from build123d import *

# Parameters (mm, degrees)
SKETCH_1_W             = 40
SKETCH_1_H             = 62
EXTRUDE_1_DEPTH        = 1
SKETCH_3_W             = 27.6
SKETCH_3_H             = 27.6
SKETCH_3_W_2           = 6.7
SKETCH_3_H_2           = 6.7
CUT_EXTRUDE_1_DEPTH    = 37.905284174
EXTRUDE_2_DEPTH        = 1
SKETCH_8_W             = 40
SKETCH_8_H             = 1
EXTRUDE_5_DEPTH        = 1
SKETCH_10_W            = 0.6
SKETCH_10_H            = 2
EXTRUDE_6_DEPTH        = 9
SKETCH_11_W            = 38.8
SKETCH_11_H            = 1
EXTRUDE_7_DEPTH        = 9
CUT_EXTRUDE_2_REACH    = 68.708
SKETCH_13_W            = 7.2
SKETCH_13_H            = 2.2
SKETCH_13_W_2          = 9.4
SKETCH_13_H_2          = 3.8
SKETCH_13_W_3          = 15
SKETCH_13_H_3          = 2.4
CUT_EXTRUDE_3_DEPTH    = 10
SKETCH_15_W            = 0.891909811
SKETCH_15_H            = 2.2
EXTRUDE_8_DEPTH        = 2.2
CUT_EXTRUDE_4_REACH    = 41.79
FILLET_1_R             = 0.5
FILLET_1_OF_MIRROR_1_R = 0.5


with BuildPart() as part:
    # 草图1 → 凸台-拉伸1 (new body)
    with BuildSketch(Plane.XY):
        Rectangle(SKETCH_1_W, SKETCH_1_H)
    extrude(amount=EXTRUDE_1_DEPTH)

    # 草图3 → 切除-拉伸1 (cut, through all)
    with BuildSketch(Plane.XY.offset(1)):
        with Locations((0, 2.2)):
            Rectangle(SKETCH_3_W, SKETCH_3_H)
        with Locations((-11.65, -19.65)):
            Rectangle(SKETCH_3_W_2, SKETCH_3_H_2)
        with Locations((-0.15, -19.65)):
            Rectangle(SKETCH_3_W_2, SKETCH_3_H_2)
        with Locations((11.45, -19.65)):
            Rectangle(SKETCH_3_W_2, SKETCH_3_H_2)
    extrude(amount=-CUT_EXTRUDE_1_DEPTH, mode=Mode.SUBTRACT)

    # 草图4 → 凸台-拉伸2 (add)
    with BuildSketch(Plane(origin=(0, 0, 0), x_dir=(-1, 0, 0), z_dir=(0, 0, -1))):
        Polygon((-16.9, 22.527428343), (-16.2, 22.527428343), (-16.2, -13.6), (16.2, -13.6), (16.2, 22.527428343), (16.9, 22.527428343), (16.9, -14.3), (15.9, -14.3), (-15.9, -14.3), (-16.9, -14.3), align=None)
    extrude(amount=EXTRUDE_2_DEPTH)

    # 草图8 → 凸台-拉伸5 (add)
    with BuildSketch(Plane.XZ.offset(31)):
        with Locations((0, 0.5)):
            Rectangle(SKETCH_8_W, SKETCH_8_H)
    extrude(amount=EXTRUDE_5_DEPTH)

    # 草图10 → 凸台-拉伸6 (add)
    with BuildSketch(Plane(origin=(0, 0, 0), x_dir=(-1, 0, 0), z_dir=(0, 0, -1))):
        with Locations((-19.7, -31)):
            Rectangle(SKETCH_10_W, SKETCH_10_H)
        with Locations((19.7, -31)):
            Rectangle(SKETCH_10_W, SKETCH_10_H)
    extrude(amount=EXTRUDE_6_DEPTH)

    # 草图11 → 凸台-拉伸7 (add)
    with BuildSketch(Plane(origin=(0, 0, 0), x_dir=(-1, 0, 0), z_dir=(0, 0, -1))):
        with Locations((0, -31.5)):
            Rectangle(SKETCH_11_W, SKETCH_11_H)
    extrude(amount=EXTRUDE_7_DEPTH)

    # 草图13 → 切除-拉伸2 (cut, up to next)
    with BuildSketch(Plane.XZ.offset(32), mode=Mode.PRIVATE) as cut_extrude_2_sk1:
        with Locations((-14.554254311, -4.4)):
            Rectangle(SKETCH_13_W, SKETCH_13_H)
    cut_extrude_2_tool1 = extrude(cut_extrude_2_sk1.sketch, amount=-CUT_EXTRUDE_2_REACH, mode=Mode.PRIVATE) & part.part
    # 草图13 → 切除-拉伸2 (cut, up to next)
    with BuildSketch(Plane.XZ.offset(32), mode=Mode.PRIVATE) as cut_extrude_2_sk2:
        with Locations((-4.454254311, -5.1)):
            Rectangle(SKETCH_13_W_2, SKETCH_13_H_2)
    cut_extrude_2_tool2 = extrude(cut_extrude_2_sk2.sketch, amount=-CUT_EXTRUDE_2_REACH, mode=Mode.PRIVATE) & part.part
    # 草图13 → 切除-拉伸2 (cut, up to next)
    with BuildSketch(Plane.XZ.offset(32), mode=Mode.PRIVATE) as cut_extrude_2_sk3:
        with Locations((9.845745689, -4.5)):
            Rectangle(SKETCH_13_W_3, SKETCH_13_H_3)
    cut_extrude_2_tool3 = extrude(cut_extrude_2_sk3.sketch, amount=-CUT_EXTRUDE_2_REACH, mode=Mode.PRIVATE) & part.part
    add(cut_extrude_2_tool1.solids().sort_by_distance((-14.554254, -32, -4.4))[0], mode=Mode.SUBTRACT)
    add(cut_extrude_2_tool2.solids().sort_by_distance((-4.454254, -32, -5.1))[0], mode=Mode.SUBTRACT)
    add(cut_extrude_2_tool3.solids().sort_by_distance((9.845746, -32, -4.5))[0], mode=Mode.SUBTRACT)

    # 草图14 → 切除-拉伸3 (cut)
    with BuildSketch(Plane.XY.offset(1)):
        Polygon((-20, 31), (-18, 31), (18, 31), (20, 31), (20, -30), (18, -30), (18, 29), (-18, 29), (-18, -30), (-20, -30), align=None)
    extrude(amount=-CUT_EXTRUDE_3_DEPTH, mode=Mode.SUBTRACT)

    # 草图15 → 凸台-拉伸8 (add)
    with BuildSketch(Plane.ZY.offset(16.9)):
        with Locations((-0.345954906, 0.1)):
            Rectangle(SKETCH_15_W, SKETCH_15_H)
    extrude_8 = extrude(amount=EXTRUDE_8_DEPTH)

    # 草图16 → 切除-拉伸4 (cut, up to next)
    with BuildSketch(Plane(origin=(0, 1.2, 0), x_dir=(1, 0, 0), z_dir=(0, 1, 0)), mode=Mode.PRIVATE) as cut_extrude_4_sk1:
        Polygon((-16.9, 0.791909811), (-19.1, 0.345954906), (-19.1, 0.791909811), align=None)
    cut_extrude_4_tool1 = extrude(cut_extrude_4_sk1.sketch, amount=-CUT_EXTRUDE_4_REACH, mode=Mode.PRIVATE) & part.part
    cut_extrude_4 = cut_extrude_4_tool1.solids().sort_by_distance((-18.366667, 1.2, -0.643258))[0]
    add(cut_extrude_4, mode=Mode.SUBTRACT)

    # 圆角1
    fillet_1_edges = [part.edges().sort_by_distance(p)[0] for p in [
        (-19.1, 0.1, -0.345954906),
    ]]
    fillet(fillet_1_edges, radius=FILLET_1_R)

    # 镜向1: 凸台-拉伸8, 切除-拉伸4 across plane
    add(extrude_8.mirror(Plane(origin=(0, 0, 0), x_dir=(0, 0, 1), z_dir=(1, 0, 0))))
    add(cut_extrude_4.mirror(Plane(origin=(0, 0, 0), x_dir=(0, 0, 1), z_dir=(1, 0, 0))), mode=Mode.SUBTRACT)

    # 圆角1 of 镜向1
    fillet_1_of_mirror_1_edges = [part.edges().sort_by_distance(p)[0] for p in [
        (19.1, 0.1, -0.345954906),
    ]]
    fillet(fillet_1_of_mirror_1_edges, radius=FILLET_1_OF_MIRROR_1_R)


solid = part.part
For this review, take the finished solid that the model builds, in its own axes (mm). A direction names the side the tool comes from. Coordinates: 2 decimals unless noted, no trailing zeros. Write each loop counter-clockwise with the first axis right and the second up, starting at its lowest first coordinate (ties: lowest second). Pieces come first, ordered by that corner, then holes. Notation, with made-up numbers: (-31.5, 14.5) -> (10.5, 14.5) arc R19 cw to (10.5, 40.5) -> close; hole circle Ø9 at (53.25, 37.5). An arc over 180 degrees is marked (long way). Write each question's results on one line, items separated by ' | '. Start each with the question number.
1) For faces 5 (the face through (-16.4, 4.2, -1)), 6 (the face through (17, -1, 1)), 7 (the face through (-17.79, 0.12, -0.61)), 8 (the face through (17.79, 0.12, -0.61)), list the 3-axis set-ups (+Z, -Z, +X, -X, +Y, -Y) from which the entire face can be reached by the end or side of a thin tool; tool diameter is ignored.
2) Consider section C-C (x = -13). Write out the cut boundary in (y, z), plus the area to 3 significant figures.
3) Consider section B-B (z = -4). Write out the cut boundary in (x, y), plus the area to 3 significant figures.
4) Insertion check: pin 1 (2 mm diameter, centred on x = 19, z = -6, fed in from +Y); pin 2 (12 mm diameter, centred on x = -8, y = -10.5, fed in from +Z); pin 3 (1.5 mm diameter, centred on x = -11, z = -4, fed in from +Y); pin 4 (10 mm diameter, centred on x = -7, y = 7, fed in from +Z) (3 decimals). Each pin has a flat end and moves straight along its axis. Give the tip position at first contact, or say it passes through.
5) Consider section A-A (x = 7). Write out the cut boundary in (y, z).
6) The part is to be moulded in two halves that separate along X. For faces 1 (the face through (0, -31, -3)), 2 (the face through (20, -31, -4)), 3 (the face through (0.3, -31.7, -9)), 4 (the face through (4, 17, 0)), say which applies: +X half, -X half, draft (parallel to the pull), parting line (faces both ways), or undercut.
7) Consider section D-D (y = -5). Write out the cut boundary in (x, z).
8) Wall thickness on L1, parallel to Z at x = -3.5, y = 26; L2, parallel to X at y = 2, z = 0.25; L3, parallel to Y at x = 9.5, z = -7.5: over which ranges is each line inside the solid? List them lowest first. Write a range as [from, to].
Geometry says:
1) face 5: -Z, +X, -X, +Y | face 6: +Z, +X, -X, +Y, -Y | face 7: -Z, -X, +Y | face 8: -Z, +X, +Y
2) outline: (-32, -9) -> (-31, -9) -> (-31, -5.5) -> (-32, -5.5) -> close; (-32, -3.3) -> (-31, -3.3) -> (-31, 0) -> (-23, 0) -> (-23, 1) -> (-32, 1) -> close; (-16.3, 0) -> (-14.3, 0) -> (-14.3, -1) -> (-13.6, -1) -> (-13.6, 0) -> (-11.6, 0) -> (-11.6, 1) -> (-16.3, 1) -> close; (16, 0) -> (29, 0) -> (29, 1) -> (16, 1) -> close | area: 34.2 mm^2
3) outline: (-20, -32) -> (-18.15, -32) -> (-18.15, -31) -> (-19.4, -31) -> (-19.4, -30) -> (-20, -30) -> close; (-10.95, -32) -> (-9.15, -32) -> (-9.15, -31) -> (-10.95, -31) -> close; (0.25, -32) -> (2.35, -32) -> (2.35, -31) -> (0.25, -31) -> close; (17.35, -32) -> (20, -32) -> (20, -30) -> (19.4, -30) -> (19.4, -31) -> (17.35, -31) -> close | area: 9.60 mm^2
4) pin 1: y = -30 | pin 2: z = 1 | pin 3: y = -31 | pin 4: through
5) outline: (-32, -9) -> (-31, -9) -> (-31, -5.7) -> (-32, -5.7) -> close; (-32, -3.3) -> (-31, -3.3) -> (-31, 0) -> (-14.3, 0) -> (-14.3, -1) -> (-13.6, -1) -> (-13.6, 0) -> (-11.6, 0) -> (-11.6, 1) -> (-32, 1) -> close; (16, 0) -> (29, 0) -> (29, 1) -> (16, 1) -> close
6) face 1: undercut | face 2: +X half | face 3: draft | face 4: undercut
7) outline: (-18, 0) -> (-16.9, 0) -> (-16.9, -1) -> (-16.2, -1) -> (-16.2, 0) -> (-13.8, 0) -> (-13.8, 1) -> (-18, 1) -> close; (13.8, 0) -> (16.2, 0) -> (16.2, -1) -> (16.9, -1) -> (16.9, 0) -> (18, 0) -> (18, 1) -> (13.8, 1) -> close
8) L1: [0, 1] | L2: [-18, -13.8], [13.8, 18] | L3: [-32, -31]
